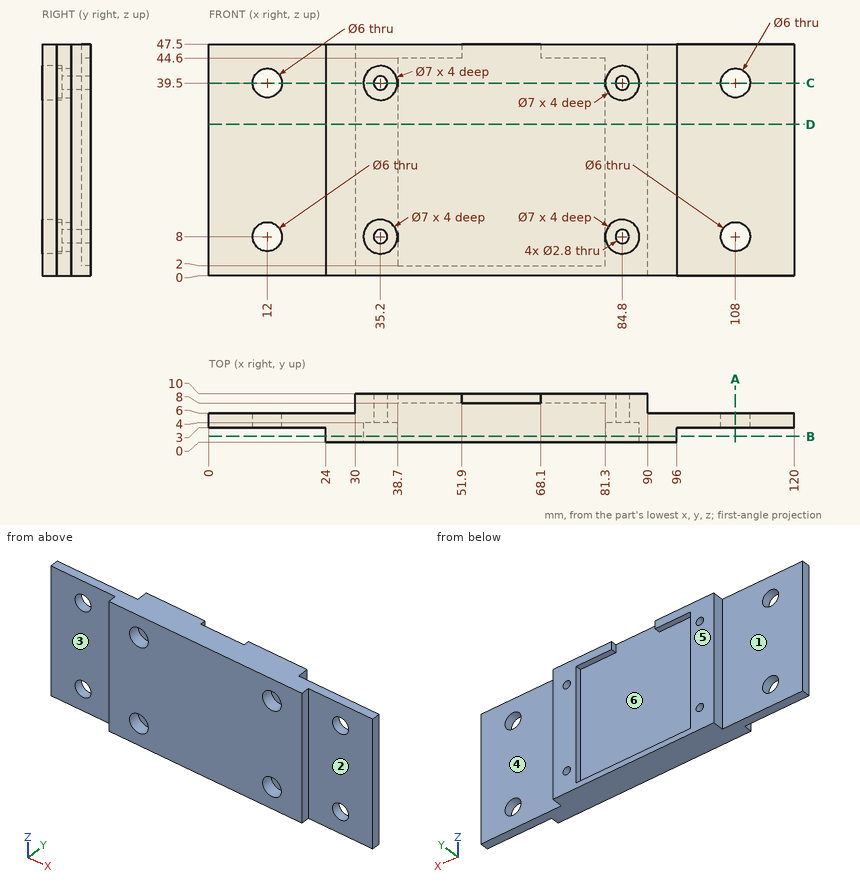
Answer from the drawing. Dimensions are ordinates in mm from the lowest x, y and z of the part. A direction names the side the tool comes from. Give positions to 0.01 mm unless a question says otherwise; leave off trailing zeros. Loops run counter-clockwise (first coordinate to the right, second up) from the corner with the lowest first, then second, coordinate; pieces in that order, holes last.
Item 1: The part is cut by section B-B (y = 1.25). Write down the section's boundary in (x, z).
Item 2: The mould has two halves that part along X. Classify the marked faces 5 and 6: released by +X, released by -X, zero draft, split by the parting line, or undercut.
Item 3: The part is cut by section C-C (z = 39.5). Give the number of separate pieces and of enclosed holes in the cut face, and give its area (3 significant figures).
Item 4: The part is cut by section A-A (x = 108). Write down the section's boundary in (y, z), and give its area (4 significant figures).
Item 5: The part is cut by section D-D (z = 31). Write down the section's boundary in (x, y).
Item 6: Each of these flat-tipped pins is pushed along its axis until it touches: pin 1 Ø1.5 at (y, z) = (1.5, 28.5) entering from -X; pin 2 Ø6 at (x, z) = (42, 41.5) entering from +Y; pin 3 Ø3 at (x, z) = (94, 15) entering from +Y. Where does it stop, or does it pass through?
Item 7: Find the intervals of material crossed by line 1 along X through (y, z) = (6.3, 39.5); line 2 along Z through (x, y) = (84.8, 5.5); line 3 along Z through (x, y) = (84.8, 2.7), in increasing order.
Item 8: For the marked faces 1, 2, 3 and 4, determine the directions among +Z, -Z, +X, -X, +Y, -Y from which every point of the face is accessible in a straight line to the end or side of a thin tool.
Taken from the geometry:
1. outline: (24, 0) - (96, 0) - (96, 47.5) - (24, 47.5) - close; hole circle Ø7 at (35.2, 8); hole circle Ø7 at (35.2, 39.5); hole circle Ø7 at (84.8, 8); hole circle Ø7 at (84.8, 39.5)
2. face 5: zero draft
2. face 6: undercut
3. separate pieces: 5
3. enclosed holes: 0
3. area: 605 mm2
4. outline: (3, 0) - (6, 0) - (6, 5) - (3, 5) - close; (3, 11) - (6, 11) - (6, 36.5) - (3, 36.5) - close; (3, 42.5) - (6, 42.5) - (6, 47.5) - (3, 47.5) - close
4. area: 106.5 mm2
5. outline: (0, 3) - (24, 3) - (24, 0) - (96, 0) - (96, 3) - (120, 3) - (120, 6) - (90, 6) - (90, 10) - (81.3, 10) - (81.3, 8) - (38.7, 8) - (38.7, 10) - (30, 10) - (30, 6) - (0, 6) - close
6. pin 1: stops at x = 24
6. pin 2: stops at y = 8
6. pin 3: stops at y = 6
7. line 1: x = 30 to 33.8, 36.6 to 83.4, 86.2 to 90
7. line 2: z = 0 to 6.6, 9.4 to 38.1, 40.9 to 47.5
7. line 3: z = 0 to 4.5, 11.5 to 36, 43 to 47.5
8. face 1: +Z, -Z, -X, +Y
8. face 2: +Z, -Z, +X, -Y
8. face 3: +Z, -Z, -X, -Y
8. face 4: +Z, -Z, +X, +Y
